Autodesk Inventor part; units mm, degrees
ref_plane "YZ Plane" through (0, 0, 0) normal (1, 0, 0) x (0, 1, 0)
ref_plane "XZ Plane" through (0, 0, 0) normal (0, 1, 0) x (-1, 0, 0)
ref_plane "XY Plane" through (0, 0, 0) normal (0, 0, 1) x (1, 0, 0)
sketch "Sketch1" plane through (0, 0, 0) normal (0, 0, 1) x (1, 0, 0)
  line L0 (0, 0) -> (400, 0)
  line L1 (400, 0) -> (400, -25.375)
  line L2 (0, -38.2) -> (12.55, -50.75)
  line L3 (400, -25.375) -> (374.625, -50.75)
  line L4 (0, -38.2) -> (0, 0)
  line L5 (374.625, -50.75) -> (12.55, -50.75)
  circle A0 centre (9, -9) radius 4
  circle A1 centre (9, -29.2) radius 4
  circle A2 centre (67.2, -9) radius 4
  circle A3 centre (67.2, -29.2) radius 4
  dimension "d3" = 8
  dimension "d4" = 8
  dimension "d5" = 8
  dimension "d6" = 8
  dimension "d10" = 9
  dimension "d11" = 9
  dimension "d12" = 9
  dimension "d13" = 9
  dimension "d15" = 20.2
  dimension "d16" = 58.2
  dimension "d18" = 12.55
  dimension "d19" = 400
  dimension "d20" = 50.75
  dimension "d21" = 25.375
  dimension "d22" = 20.2
  dimension "d23" = 58.2
  dimension "d24" = 12.55
  dimension "d25" = 25.375
extrude "Extrusion1" add sketch "Sketch1" along normal blind 3.1
properties part number "SideBracket" material "Steel, Mild"
Read the model definition and answer for the solid it produces. Units are mm, in the model's axes. Give positions to 0.01 mm unless a question says otherwise; leave off trailing zeros. Write each loop counter-clockwise with the first axis right and the second up, starting at its lowest first coordinate (ties: lowest second). Pieces come first, ordered by that corner, then holes. Notation, with made-up numbers: (86.25, 55) - (97.25, 55) arc R28 ccw to (97.25, 84) - close; hole circle Ø8 at (3, 34.5). An arc over 180 degrees is marked (long way). Use CSV: the item, a comma, the result in double quotes. Start each with the question number.
Item 1: The part is cut by section D-D, the plane y = -43.5. Give the vertices of the cut face in (x, z) (3 decimals).
Item 2: The mould has two halves that part along X. Classify faces 1 (the flat face through (197, -25, 0)), 2 (the flat face through (387.49, -37.885, 1.528)), 3 (the cylindrical face through (5, -9, 2)), 4 (the cylindrical face through (64.25, -31.9, 1.53)): pulls with the +X half, pulls with the -X half, needs draft (parallel to the pull), parting line crosses it, or undercut.
Item 3: The part is cut by section B-B, the plane y = -9. Give the vertices of the cut face in (x, z).
Item 4: Consider line 1 (Y direction, x = 67.2, z = 2.3); line 2 (X direction, y = -5.5, z = 2.25); line 3 (X direction, y = -28.5, z = 1.2) (3 decimals). Determine where each line is inside the solid, lowest interval first.
Item 5: The part is cut by section C-C, the plane z = 0.75. Give the vertices of the cut face in (x, y) (3 decimals).
Item 6: The part is cut by section A-A, the plane x = 67.2. Give the vertices of the cut face in (y, z).
Taken from the geometry:
1,outline,"(5.3, 0) - (381.875, 0) - (381.875, 3.1) - (5.3, 3.1) - close"
2,face 1,"needs draft"
2,face 2,"pulls with the +X half"
2,face 3,"undercut"
2,face 4,"undercut"
3,outline,"(0, 0) - (5, 0) - (5, 3.1) - (0, 3.1) - close; (13, 0) - (63.2, 0) - (63.2, 3.1) - (13, 3.1) - close; (71.2, 0) - (400, 0) - (400, 3.1) - (71.2, 3.1) - close"
4,line 1,"-50.75 to -33.2, -25.2 to -13, -5 to 0"
4,line 2,"0 to 7.06, 10.94 to 65.26, 69.14 to 400"
4,line 3,"0 to 5.062, 12.938 to 63.262, 71.138 to 396.875"
5,outline,"(0, -38.2) - (12.55, -50.75) - (374.625, -50.75) - (400, -25.375) - (400, 0) - (0, 0) - close; hole circle Ø8 at (9, -29.2); hole circle Ø8 at (9, -9); hole circle Ø8 at (67.2, -29.2); hole circle Ø8 at (67.2, -9)"
6,outline,"(-50.75, 0) - (-33.2, 0) - (-33.2, 3.1) - (-50.75, 3.1) - close; (-25.2, 0) - (-13, 0) - (-13, 3.1) - (-25.2, 3.1) - close; (-5, 0) - (0, 0) - (0, 3.1) - (-5, 3.1) - close"
